Geometry: see drawing. Coordinates: mm, zero at the bounding-box minimum. A direction names the side the tool comes from. Coordinates: 2 decimals unless noted, no trailing zeros. Write each loop counter-clockwise with the first axis right and the second up, starting at its lowest first coordinate (ties: lowest second). Pieces come first, ordered by that corner, then holes. Notation, with made-up numbers: (36.5, -10.5) -> (82.5, -10.5) arc R26 cw to (82.5, 3.5) -> close; hole circle Ø7 at (1.5, -14). An arc over 180 degrees is marked (long way). Answer as a JSON object with one key per item and string values. Group by question number.
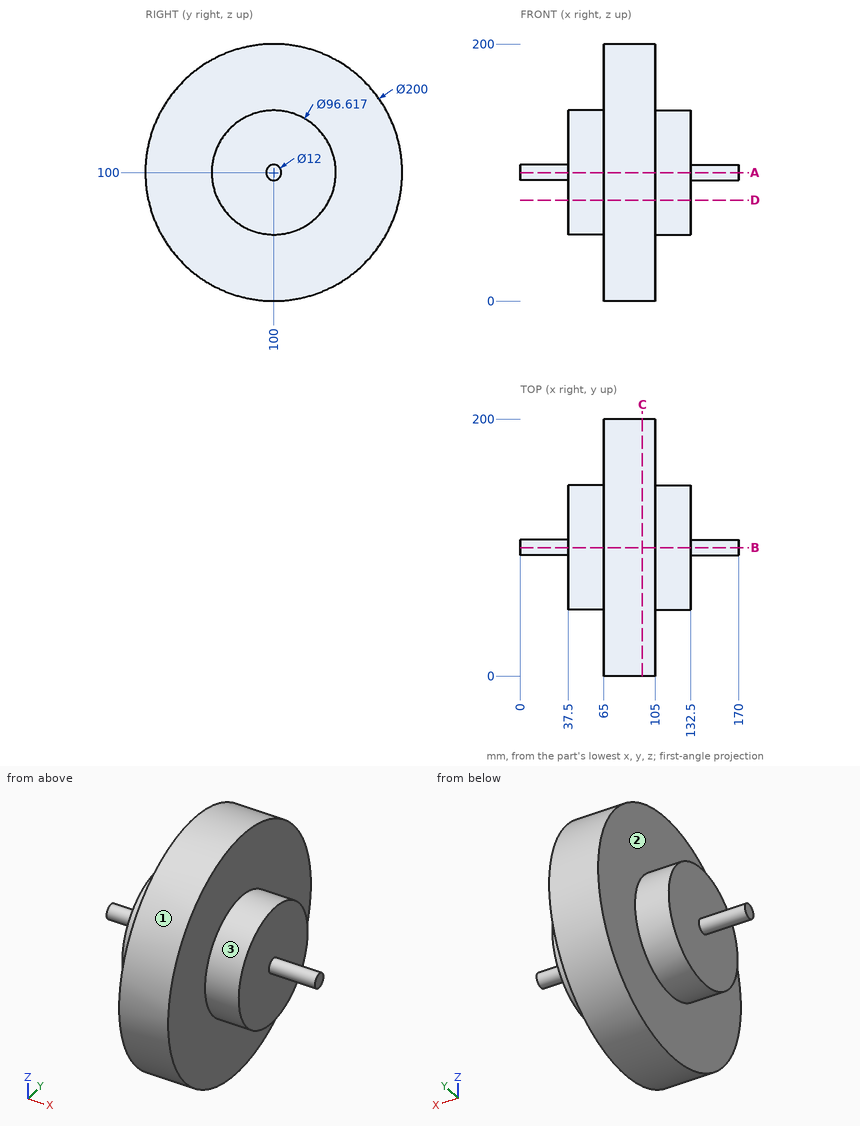
Item 1: Section C-C on x = 95. Output: boundary loops of the cut face in (y, z).
Item 2: Section D-D on z = 78.5. Output: boundary loops of the cut face in (x, y), then the cut area to 3 significant figures.
Item 3: Contact query for flat-ended pins moving along their axis: pin 1 (12 mm diameter, centred on x = 67, z = 141, fed in from -Y) (1 decimal); pin 2 (1 mm diameter, centred on y = 97.5, z = 113, fed in from +X); pin 3 (1.5 mm diameter, centred on x = 85.5, z = 127.5, fed in from +Y). Output: stop coordinate, or through.
Item 4: Set-up query: the marked faces 1, 2 and 3. Return all of +Z, -Z, +X, -X, +Y, -Y with unobstructed straight access to the full face (end or side cutting, diameter ignored); none if empty.
Item 5: Ray query, L1, parallel to X at y = 101, z = 58.5; L2, parallel to X at y = 69, z = 38; L3, parallel to Y at x = 66, z = 58. Return the intervals inside material, ascending. Write a range as [from, to].
Item 6: Section A-A on z = 100. Output: boundary loops of the cut face in (x, y), then the cut area to 3 significant figures.
Answer sheet:
{
 "1": {"outline": "circle Ø200 at (100, 100)"},
 "2": {"outline": "(37.5, 56.74) -> (65, 56.74) -> (65, 2.34) -> (105, 2.34) -> (105, 56.74) -> (132.5, 56.74) -> (132.5, 143.26) -> (105, 143.26) -> (105, 197.66) -> (65, 197.66) -> (65, 143.26) -> (37.5, 143.26) -> close", "area": "12,600 mm^2"},
 "3": {"pin 1": "stops at y = 6.3", "pin 2": "stops at x = 132.5", "pin 3": "stops at y = 196.36"},
 "4": {"face 1": "+X, -X", "face 2": "-X", "face 3": "+X"},
 "5": {"L1": "x = [37.5, 132.5]", "L2": "x = [65, 105]", "L3": "y = [9.25, 190.75]"},
 "6": {"outline": "(0, 94) -> (37.5, 94) -> (37.5, 51.69) -> (65, 51.69) -> (65, 0) -> (105, 0) -> (105, 51.69) -> (132.5, 51.69) -> (132.5, 94) -> (170, 94) -> (170, 106) -> (132.5, 106) -> (132.5, 148.31) -> (105, 148.31) -> (105, 200) -> (65, 200) -> (65, 148.31) -> (37.5, 148.31) -> (37.5, 106) -> (0, 106) -> close", "area": "14,200 mm^2"}
}
